```python
from build123d import *

# Parameters (mm, degrees)
BOSS_EXTRUDE1_DEPTH = 4
SKETCH2_R           = 3.5
SKETCH2_R_2         = 3.302
CUT_EXTRUDE1_DEPTH  = 378.918311279
SKETCH5_R           = 3
CUT_EXTRUDE2_DEPTH  = 378.918311279


with BuildPart() as part:
    # Sketch1 → Boss-Extrude1 (new body)
    with BuildSketch(Plane.XY):
        with BuildLine():
            Line((-350, 122.5), (350, 122.5))
            Line((350, 122.5), (350, -122.5))
            Line((350, -122.5), (320, -122.5))
            ThreePointArc((320, -122.5), (316.464466094, -123.964466094), (315, -127.5))
            Line((315, -127.5), (315, -137.5))
            ThreePointArc((315, -137.5), (313.535533906, -141.035533906), (310, -142.5))
            Line((310, -142.5), (193.06, -142.5))
            ThreePointArc((193.06, -142.5), (189.524466094, -141.035533906), (188.06, -137.5))
            Line((188.06, -137.5), (188.06, -127.5))
            ThreePointArc((188.06, -127.5), (186.595533906, -123.964466094), (183.06, -122.5))
            Line((183.06, -122.5), (-183.06, -122.5))
            ThreePointArc((-183.06, -122.5), (-186.595533906, -123.964466094), (-188.06, -127.5))
            Line((-188.06, -127.5), (-188.06, -137.5))
            ThreePointArc((-188.06, -137.5), (-189.524466094, -141.035533906), (-193.06, -142.5))
            Line((-193.06, -142.5), (-310, -142.5))
            ThreePointArc((-310, -142.5), (-313.535533906, -141.035533906), (-315, -137.5))
            Line((-315, -137.5), (-315, -127.5))
            ThreePointArc((-315, -127.5), (-316.464466094, -123.964466094), (-320, -122.5))
            Line((-320, -122.5), (-350, -122.5))
            Line((-350, -122.5), (-350, 122.5))
        make_face()
    extrude(amount=BOSS_EXTRUDE1_DEPTH)

    # Sketch2 → Cut-Extrude1 (cut, through all)
    with BuildSketch(Plane.XY.offset(4)):
        with Locations((-299.029618848, -97.636758765)):
            Circle(SKETCH2_R)
        with Locations((-204.029618848, -97.636758765)):
            Circle(SKETCH2_R)
        with Locations((-289.030381152, -125.636758765)):
            Circle(SKETCH2_R_2)
        with Locations((-214.030381152, -125.636758765)):
            Circle(SKETCH2_R_2)
        with Locations((204.02961885, -97.636758765)):
            Circle(SKETCH2_R)
        with Locations((299.02961885, -97.636758765)):
            Circle(SKETCH2_R)
        with Locations((214.028856546, -125.636758765)):
            Circle(SKETCH2_R_2)
        with Locations((289.028856546, -125.636758765)):
            Circle(SKETCH2_R_2)
        with BuildLine():
            ThreePointArc((-235.273778228, -91.777635644), (-251.529618848, 7.973241235), (-267.785459469, -91.777635644))
            ThreePointArc((-267.785459469, -91.777635644), (-251.529618848, -102.696758765), (-235.273778228, -91.777635644))
        make_face()
        with BuildLine():
            ThreePointArc((267.78545947, -91.777635644), (251.52961885, 7.973241235), (235.27377823, -91.777635644))
            ThreePointArc((235.27377823, -91.777635644), (251.52961885, -102.696758765), (267.78545947, -91.777635644))
        make_face()
    extrude(amount=-CUT_EXTRUDE1_DEPTH, mode=Mode.SUBTRACT)

    # Sketch5 → Cut-Extrude2 (cut, through all)
    with BuildSketch(Plane.XY.offset(4)):
        with Locations((-340, -107.5)):
            Circle(SKETCH5_R)
        with Locations((-340, 112.5)):
            Circle(SKETCH5_R)
        with Locations((-171, 112.5)):
            Circle(SKETCH5_R)
        with Locations((-171, -107.5)):
            Circle(SKETCH5_R)
        with Locations((171, -107.5)):
            Circle(SKETCH5_R)
        with Locations((340, 112.5)):
            Circle(SKETCH5_R)
        with Locations((340, -107.5)):
            Circle(SKETCH5_R)
        with Locations((171, 112.5)):
            Circle(SKETCH5_R)
        with Locations((25, 112.5)):
            Circle(SKETCH5_R)
        with Locations((25, -107.5)):
            Circle(SKETCH5_R)
        with Locations((-255.5, 112.5)):
            Circle(SKETCH5_R)
        with Locations((98, 112.5)):
            Circle(SKETCH5_R)
        with Locations((255.5, 112.5)):
            Circle(SKETCH5_R)
        with Locations((340, 2.25)):
            Circle(SKETCH5_R)
        with Locations((171, 2)):
            Circle(SKETCH5_R)
        with Locations((25, 2.25)):
            Circle(SKETCH5_R)
        with Locations((-171, 2.25)):
            Circle(SKETCH5_R)
        with Locations((-340, 2.25)):
            Circle(SKETCH5_R)
        with Locations((-73, 112.5)):
            Circle(SKETCH5_R)
        with Locations((-73, -107.5)):
            Circle(SKETCH5_R)
        with Locations((-325, -107.5)):
            Circle(SKETCH5_R)
        with Locations((186, -107.5)):
            Circle(SKETCH5_R)
        with Locations((325, -107.5)):
            Circle(SKETCH5_R)
        with Locations((-186, -107.5)):
            Circle(SKETCH5_R)
        with Locations((98, -107.5)):
            Circle(SKETCH5_R)
    extrude(amount=-CUT_EXTRUDE2_DEPTH, mode=Mode.SUBTRACT)


solid = part.part
```
Geometry: final body of the model. Coordinates: model frame, mm. Coordinates: 2 decimals unless noted, no trailing zeros. Order: outer loops, then holes, each group sorted by start corner. A loop starts at its lowest first (then second) coordinate and runs counter-clockwise, first axis right, second up. Notation, with made-up numbers: (-9.75, 66) -> (39.25, 66) arc R30 cw to (39.25, 95) -> close; hole circle Ø8 at (61, 63). An arc over 180 degrees is marked (long way). Answer in a Markdown table with one row per item.
Item 1: Contact query for a flat-ended pin moving along its axis: P1, Ø5.5, axis at x = -214.03, y = -125.64, coming from the +Z side. Output: stop coordinate, or through.
Return value:
| item | result |
|---|---|
| P1 | passes through |
Item 2: Draft query along Y for faces 1 (the cylindrical face through (-249.51, 7.933, 2.028)), 2 (the cylindrical face through (253.549, 7.933, 2.028)), 3 (the flat face through (5, -8, 4)). Return one class per face: released by +Y, released by -Y, zero draft, split by the parting line, or undercut.
Return value:
| item | result |
|---|---|
| face 1 | undercut |
| face 2 | undercut |
| face 3 | zero draft |
Item 3: Section C-C on z = 2.85. State how many separate pieces and enclosed holes the cut face has, plus the area to 3 significant figures.
Return value:
| item | result |
|---|---|
| separate pieces | 1 |
| enclosed holes | 35 |
| area | 159,000 mm² |
Item 4: Ray query, L1, parallel to Y at x = -171, z = 2.75; L2, parallel to Y at x = -255.5, z = 1.15; L3, parallel to X at y = -62, z = 2.6. Return the intervals inside material, ascending.
Return value:
| item | result |
|---|---|
| L1 | y = -122.5 to -110.5, -104.5 to -0.75, 5.25 to 109.5, 115.5 to 122.5 |
| L2 | y = -142.5 to -102.24, 7.82 to 109.5, 115.5 to 122.5 |
| L3 | x = -350 to -299.16, -203.9 to 203.9, 299.16 to 350 |
Item 5: Section B-B on x = 124.5. Output: boundary loops of the cut face in (y, z), plus the area to 3 significant figures.
Return value:
| item | result |
|---|---|
| outline | (-122.5, 0) -> (122.5, 0) -> (122.5, 4) -> (-122.5, 4) -> close |
| area | 980 mm² |
Item 6: Section A-A on y = -65.5. Output: boundary loops of the cut face in (x, z).
Return value:
| item | result |
|---|---|
| outline | (-350, 0) -> (-297.63, 0) -> (-297.63, 4) -> (-350, 4) -> close; (-205.43, 0) -> (205.43, 0) -> (205.43, 4) -> (-205.43, 4) -> close; (297.63, 0) -> (350, 0) -> (350, 4) -> (297.63, 4) -> close |
